For this review, take the finished solid that the model builds, in its own axes (mm). Face numbers are marked on the shaded views. A direction names the side the tool comes from. Give positions to 0.01 mm unless a question says otherwise; leave off trailing zeros. Write each loop counter-clockwise with the first axis right and the second up, starting at its lowest first coordinate (ties: lowest second). Pieces come first, ordered by that corner, then holes. Notation, with made-up numbers: M 45,63 L 57,63 A12 cw 57,77 Z; hole C 1.25,71 d6. An arc over 180 degrees is marked long. Write item = value, one per line.
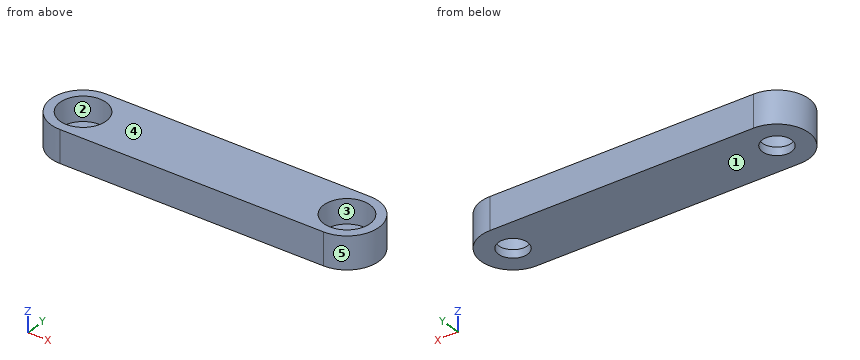
Solid Edge part; units mm, degrees
sketch "Sketch1" plane through (0, 0, 0) normal (0, 0, 1) x (1, 0, 0)
  arc A0 (16, 3.95) -> (16, -3.95) centre (16, 0) cw
  line L0 (16, -3.95) -> (-16, -3.95)
  arc A1 (-16, 3.95) -> (-16, -3.95) centre (-16, 0) ccw
  line L1 (16, 3.95) -> (-16, 3.95)
extrude "Protrusion1" add sketch "Sketch1" along normal blind 4
hole "Hole_3" at (-16, 0, 4) direction (0, 0, -1) diameter 3.6 end up to next
hole "Hole1" at (16, 0, 4) direction (0, 0, -1) diameter 3.6 end up to next
hole "Hole_5" at (-16, 0, 4) direction (0, 0, -1) diameter 5.7 depth 3
hole "Hole2" at (16, 0, 4) direction (0, 0, -1) diameter 5.7 depth 3
1. We need section A-A, the plane y = 0. Write out the cut boundary in (x, z), then the cut area to 3 significant figures.
Responses:
outline = M -19.95,0 L -17.8,0 L -17.8,1 L -18.85,1 L -18.85,4 L -19.95,4 Z; M -14.2,0 L 14.2,0 L 14.2,1 L 13.15,1 L 13.15,4 L -13.15,4 L -13.15,1 L -14.2,1 Z; M 17.8,0 L 19.95,0 L 19.95,4 L 18.85,4 L 18.85,1 L 17.8,1 Z
area = 118 mm2
2. Machinability: for the marked faces 1 and 2, which of the approach directions +Z, -Z, +X, -X, +Y, -Y give a long, thin tool a straight path to every point of the face, cutting with its end or side? Answer none if there is none.
Responses:
face_1 = -Z, +X, -X, +Y, -Y
face_2 = +Z
3. We need section B-B, the plane z = 3.6. Write out the cut boundary in (x, y), then the cut area to 3 significant figures.
Responses:
outline = M -16,-3.95 L 16,-3.95 A3.95 ccw 16,3.95 L -16,3.95 A3.95 ccw Z; hole C -16,0 d5.7; hole C 16,0 d5.7
area = 251 mm2
4. For line 1 along X through (y, z) = (0, 0.8); line 2 along X through (y, z) = (0, 3.45); line 3 along Y through (x, z) = (-16, 1.85), list the stretches that pass through material, from the lowest coordinate up. Write a range as from..to.
Responses:
line_1 = -19.95..-17.8, -14.2..14.2, 17.8..19.95
line_2 = -19.95..-18.85, -13.15..13.15, 18.85..19.95
line_3 = -3.95..-2.85, 2.85..3.95
5. The part is to be moulded in two halves that separate along X. For the marked faces 3, 4 and 5, say which applies: +X half, -X half, draft (parallel to the pull), parting line (faces both ways), or undercut.
Responses:
face_3 = undercut
face_4 = draft
face_5 = +X half
6. Insertion check: P1, Ø3, axis at x = -15, y = -0.5, coming from the +Z side. The pin has a flat end and moves straight along its axis. Give the tip position at first contact, or say it passes through.
Responses:
P1 = 1
